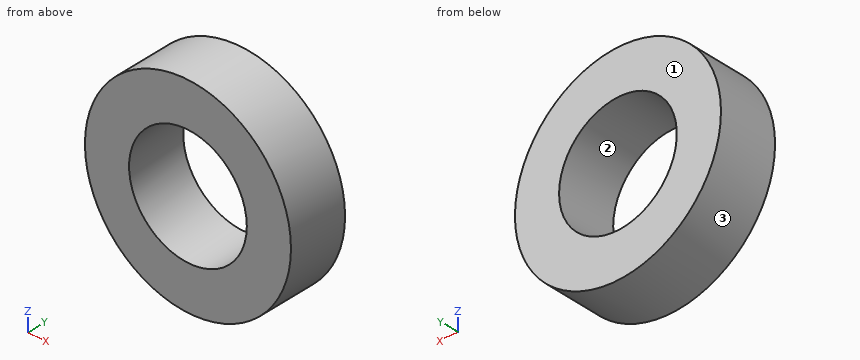
from build123d import *

# Parameters (mm, degrees)
F0_R     = 4
F1_DEPTH = 4.5
F0_R_2   = 7
F2_DEPTH = 4


with BuildPart() as f1:
    # F0 (on Front) → F1 (new body)
    with BuildSketch(Plane.XZ):
        with Locations((0.566548, 0)):
            Circle(F0_R)
    extrude(amount=-F1_DEPTH)


with BuildPart() as f2:
    # F0 (on Front) → F2 (new body)
    with BuildSketch(Plane.XZ):
        with Locations((0.566548, 0)):
            Circle(F0_R_2)
        with Locations((0.566548, 0)):
            Circle(F0_R, mode=Mode.SUBTRACT)
    extrude(amount=-F2_DEPTH)


solid = f2.part
Verification items for the finished model (mm, model axes). Face numbers are marked on the shaded views. Give positions to 0.01 mm unless a question says otherwise; leave off trailing zeros. Loops run counter-clockwise (first coordinate to the right, second up) from the corner with the lowest first, then second, coordinate; pieces in that order, holes last.
1) Draft check along X on the marked faces 1, 2 and 3. Enter one of: pulls with the +X half, pulls with the -X half, needs draft (parallel to the pull), parting line crosses it, or undercut.
2) Sectioned sample at C-C, the plane y = 2.55. Enter the section's corners in (x, z), then the cut area to 3 significant figures.
3) Sectioned sample at A-A, the plane z = 0. Enter the section's corners in (x, y), then the cut area to 3 significant figures.
4) Depth check by flat-ended pin: pin 1 Ø1 at (x, y) = (5, 2.5) entering from -Z; pin 2 Ø5 at (x, z) = (0.57, 0) entering from -Y; pin 3 Ø2 at (x, z) = (4, 1.5) entering from +Y; pin 4 Ø2 at (y, z) = (3.5, -4.5) entering from +X. Enter the tip coordinate at first touch or a pass-through.
5) Sectioned sample at B-B, the plane x = -1.5. Enter the section's corners in (y, z), then the cut area to 3 significant figures.
6) Sectioned sample at D-D, the plane z = 6. Enter the section's corners in (x, y), then the cut area to 3 significant figures.
7) Thickness scan on line 1 along Z through (x, y) = (0.5, 1.3); line 2 along X through (y, z) = (0.7, -2.25); line 3 along Z through (x, y) = (4.25, 0.95). Record the ranges inside material, lowest first.
Answers:
1. face 1: needs draft
1. face 2: undercut
1. face 3: parting line crosses it
2. outline: circle Ø14 at (0.57, 0); hole circle Ø8 at (0.57, 0)
2. area: 104 mm2
3. outline: (-6.43, 0) - (-3.43, 0) - (-3.43, 4) - (-6.43, 4) - close; (4.57, 0) - (7.57, 0) - (7.57, 4) - (4.57, 4) - close
3. area: 24.0 mm2
4. pin 1: stops at z = -5.79
4. pin 2: passes through
4. pin 3: stops at y = 4
4. pin 4: stops at x = 6.63
5. outline: (0, -6.69) - (4, -6.69) - (4, -3.42) - (0, -3.42) - close; (0, 3.42) - (4, 3.42) - (4, 6.69) - (0, 6.69) - close
5. area: 26.1 mm2
6. outline: (-3.04, 0) - (4.17, 0) - (4.17, 4) - (-3.04, 4) - close
6. area: 28.8 mm2
7. line 1: z = -7 to -4, 4 to 7
7. line 2: x = -6.06 to -2.74, 3.87 to 7.2
7. line 3: z = -5.95 to -1.56, 1.56 to 5.95
